The model under review builds one solid part; all positions refer to its coordinate system, in mm. Face numbers are marked on the shaded views. Coordinates: 2 decimals unless noted, no trailing zeros. Order: outer loops, then holes, each group sorted by start corner. A loop starts at its lowest first (then second) coordinate and runs counter-clockwise, first axis right, second up. Notation, with made-up numbers: (2, 41.25) - (35, 41.25) arc R22 ccw to (35, 80.25) - close; hole circle Ø4 at (60.5, -27.75). An arc over 180 degrees is marked (long way). Answer in a Markdown table with one row per item.
Autodesk Inventor part; units mm, degrees
ref_plane "YZ Plane" through (0, 0, 0) normal (1, 0, 0) x (0, 1, 0)
ref_plane "XZ Plane" through (0, 0, 0) normal (0, 1, 0) x (-1, 0, 0)
ref_plane "XY Plane" through (0, 0, 0) normal (0, 0, 1) x (1, 0, 0)
sketch "スケッチ1" plane through (0, 0, 0) normal (1, 0, 0) x (0, 1, 0)
  line L0 (0, 0) -> (15, 0) construction
  line L1 (15, 0) -> (15, -10) construction
  line L2 (15, -10) -> (16, -10)
  line L3 (16, -10) -> (16, 10)
  line L4 (16, 10) -> (15, 10)
  line L5 (15, 10) -> (15, -10)
  line L6 (0, -14) -> (0, 14)
  dimension "d0" = 15
  dimension "d2" = 1
  dimension "d3" = 20
revolve "回転1" add sketch "スケッチ1" angle 180 about axis through (0, 0, -10) along (0, 0, 1)
sketch "スケッチ2" plane through (0, 15, 10) normal (1, 0, 0) x (0, 0, -1)
  line L0 (20, 1) -> (0, 1)
  line L1 (0, 1) -> (3, 1)
  line L2 (3, 1) -> (11, 1)
  line L3 (11, 1) -> (11, -6)
  line L4 (11, -6) -> (3, -6)
  line L5 (3, -6) -> (3, 1)
  point P0 (10, -15)
  dimension "d6" = 8
  dimension "d7" = 7
extrude "押し出し1" cut sketch "スケッチ2" against normal through all
properties part number "cover-pipe" material "ステンレス鋼"
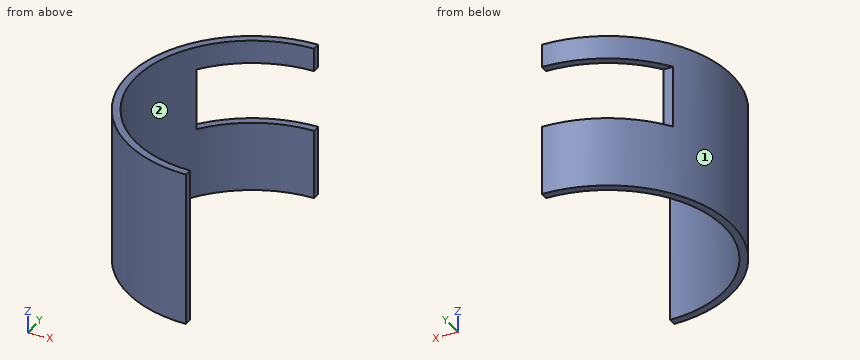
Item 1: We need section C-C, the plane z = -4.75. Write out the cut boundary in (x, y), then the cut area to 3 significant figures.
Check values:
| item | result |
|---|---|
| outline | (0, -16) - (0, -15) arc R15 cw to (0, 15) - (0, 16) arc R16 ccw to start |
| area | 48.7 mm^2 |
Item 2: We need section A-A, the plane x = -9.75. Write out the cut boundary in (y, z).
Check values:
| item | result |
|---|---|
| outline | (-12.69, -10) - (-11.4, -10) - (-11.4, 10) - (-12.69, 10) - close; (11.4, -10) - (12.69, -10) - (12.69, -1) - (11.4, -1) - close; (11.4, 7) - (12.69, 7) - (12.69, 10) - (11.4, 10) - close |
Item 3: Clearance check with flat-ended pins moving along their axes: pin 1 Ø0.6 at (x, z) = (-12.5, 2) entering from +Y; pin 2 Ø4 at (y, z) = (2.5, 7.5) entering from -X. State where each tip first meets the part, or that it passes through.
Check values:
| item | result |
|---|---|
| pin 1 | y = 9 |
| pin 2 | x = -15.99 |
Item 4: We need section B-B, the plane y = 12. Write out the cut boundary in (x, z).
Check values:
| item | result |
|---|---|
| outline | (-10.58, -10) - (-9, -10) - (-9, -1) - (-10.58, -1) - close; (-10.58, 7) - (-9, 7) - (-9, 10) - (-10.58, 10) - close |
Item 5: We need section D-D, the plane x = -2. Write out the cut boundary in (y, z).
Check values:
| item | result |
|---|---|
| outline | (-15.87, -10) - (-14.87, -10) - (-14.87, 10) - (-15.87, 10) - close; (14.87, -10) - (15.87, -10) - (15.87, -1) - (14.87, -1) - close; (14.87, 7) - (15.87, 7) - (15.87, 10) - (14.87, 10) - close |
Item 6: Mouldability with a two-part tool opening along Y and no side actions: class the marked faces 1 and 2 as +Y half, -Y half, draft (parallel to the pull), parting line (faces both ways), or undercut.
Check values:
| item | result |
|---|---|
| face 1 | parting line |
| face 2 | undercut |
Item 7: To check wall thickness, follow line 1 (Y direction, x = -4, z = 7.5); line 2 (Y direction, x = -9.25, z = 9.25); line 3 (X direction, y = 0, z = 2.25). State the ranges of each line that lie inside material, in increasing order. Write a range as from..to.
Check values:
| item | result |
|---|---|
| line 1 | -15.49..-14.46, 14.46..15.49 |
| line 2 | -13.06..-11.81, 11.81..13.06 |
| line 3 | -16..-15 |
